Could you check a few things on this model? Use its own coordinates, in mm. Give positions to 0.01 mm unless a question says otherwise; leave off trailing zeros. Loops run counter-clockwise (first coordinate to the right, second up) from the corner with the lowest first, then second, coordinate; pieces in that order, holes last. Notation, with made-up numbers: (8, 40) - (15, 40) arc R27 cw to (15, 77) - close; hole circle Ø1 at (-22.5, 88). An arc over 180 degrees is marked (long way). Use CSV: the item, a comma, the result in double quotes.
Autodesk Inventor part; units mm, degrees
ref_plane "YZ Plane" through (0, 0, 0) normal (1, 0, 0) x (0, 1, 0)
ref_plane "XZ Plane" through (0, 0, 0) normal (0, 1, 0) x (-1, 0, 0)
ref_plane "XY Plane" through (0, 0, 0) normal (0, 0, 1) x (1, 0, 0)
sketch "スケッチ3" plane through (0, 0, 0) normal (0, 0, 1) x (1, 0, 0)
  line L0 (60, -99.3436) -> (-60, -99.3436)
  line L1 (-60, -99.3436) -> (-60, 99.3436)
  line L2 (-60, 99.3436) -> (60, 99.3436)
  line L3 (60, 99.3436) -> (60, -99.3436)
  line L4 (60, -99.3436) -> (-60, 99.3436) construction
  line L5 (-60, -99.3436) -> (60, 99.3436) construction
  point P0 (0, 0)
  dimension "d25" = 120
extrude "押し出し1" add sketch "スケッチ3" against normal blind 3
sketch "スケッチ4" plane through (0, 0, 0) normal (0, 0, 1) x (1, 0, 0)
  line L0 (0, 45.0711) -> (68.3595, 45.0711)
  line L1 (68.3595, 45.0711) -> (-74.3824, 45.0711)
  line L2 (-74.3824, 45.0711) -> (108.1656, 45.0711)
  line L3 (108.1656, 45.0711) -> (108.1656, 129.4154)
  line L4 (108.1656, 129.4154) -> (-74.3824, 129.4154)
  line L5 (-74.3824, 129.4154) -> (-74.3824, 45.0711)
  point P0 (0, 0)
extrude "押し出し4" cut sketch "スケッチ4" against normal blind 10
sketch "スケッチ13" plane through (0, 0, 0) normal (0, 0, 1) x (1, 0, 0)
  circle A0 centre (0, 0) radius 7.5
  circle A1 centre (0, 0) radius 32.5
  circle A2 centre (31.7707, 6.8465) radius 25
  circle A3 centre (31.7707, 6.8465) radius 7.5
  circle A4 centre (31.7707, 6.8465) radius 32.5
  circle A5 centre (28.5436, -25.4929) radius 25
  circle A6 centre (28.5436, -25.4929) radius 20
  circle A7 centre (28.5436, -25.4929) radius 60
  circle A8 centre (0, -78.2685) radius 40
  circle A9 centre (0, -78.2685) radius 50
  circle A10 centre (31.7707, 6.8465) radius 5.05
  circle A11 centre (28.5436, -25.4929) radius 9.55
  circle A12 centre (0, -78.2685) radius 9.55
  dimension "d87" = 65
  dimension "d89" = 65
  dimension "d91" = 120
  dimension "d86" = 15
  dimension "d88" = 15
  dimension "d90" = 40
  dimension "d92" = 100
  dimension "d96" = 10.1
  dimension "d97" = 19.1
  dimension "d98" = 19.1
extrude "押し出し16" cut sketch "スケッチ13" against normal blind 10 contours A10 A1 | A1 A10 | A11 A1 A2 | A2 A1 A4 A11 | A4 A1 A11 | A2 A11 A4 A1 | A1 A11 A2 | A4 A11 A1 | A12 A7 | A7 A12
sketch "スケッチ14" plane through (0, 0, 0) normal (0, 0, 1) x (1, 0, 0)
  point P0 (0, 0)
sketch "スケッチ15" plane through (0, 0, 0) normal (0, 0, 1) x (1, 0, 0)
  line L0 (-60, -99.3436) -> (-60, 45.0711)
  line L1 (60, 45.0711) -> (60, -99.3436)
  line L2 (-60, 45.0711) -> (60, 45.0711)
  line L3 (60, 45.0711) -> (60, -92.9289)
  line L4 (60, -92.9289) -> (-60, -92.9289)
  line L5 (-60, -92.9289) -> (-60, 45.0711)
  point P0 (0, 0)
  dimension "d101" = 138
extrude "押し出し17" cut sketch "スケッチ15" against normal blind 10 keep common part
sketch "スケッチ16" plane through (-60, 45.0711, 0) normal (0, 1, 0) x (1, 0, 0)
  line L0 (-11.4218, 21.1899) -> (145.405, 21.1899)
  line L1 (145.405, 21.1899) -> (145.405, -40.3361)
  line L2 (145.405, -40.3361) -> (-11.4218, -40.3361)
  line L3 (-11.4218, -40.3361) -> (-11.4218, 21.1899)
  point P0 (60, 0)
extrude "押し出し18" cut sketch "スケッチ16" against normal blind 10
sketch "スケッチ17" plane through (0, 0, 0) normal (0, 0, 1) x (1, 0, 0)
  circle A0 centre (31.7707, 6.8465) radius 5
  circle A1 centre (31.7707, 6.8465) radius 25
  circle A2 centre (28.5436, -25.4929) radius 9.5
  circle A3 centre (28.5436, -25.4929) radius 25
  circle A4 centre (55, -13) radius 2.1
  circle A5 centre (-55, -13) radius 2.1
  circle A6 centre (0, 29) radius 2.1
  point P0 (0, 0)
  point P1 (0, 0)
  dimension "d106" = 50
  dimension "d107" = 50
  dimension "d108" = 4.2
  dimension "d109" = 4.2
  dimension "d110" = 4.2
extrude "押し出し19" cut sketch "スケッチ17" against normal blind 10 contours A4 | A5 | A6
sketch "スケッチ18" plane through (0, 0, -3) normal (0, 0, -1) x (-1, 0, 0)
  circle A0 centre (52.5, -85.929) radius 1.6
  circle A1 centre (52.5, -77.929) radius 1.6
  circle A2 centre (-52.5, -77.929) radius 1.6
  circle A3 centre (-52.5, -85.929) radius 1.6
  point P0 (0, 0)
  dimension "d113" = 3.2
  dimension "d114" = 3.2
  dimension "d115" = 3.2
  dimension "d116" = 3.2
extrude "押し出し20" cut sketch "スケッチ18" against normal blind 10
fillet "フィレット2" radius 2 4 edges at (0, 35.0711, -3) (-60, 35.0711, -1.5) (-60, -92.9289, -1.5) (60, -92.9289, -1.5)
fillet "フィレット3" radius 2 8 edges at (60, 34.4853, -2.4142) (60, -28.9289, -3) (59.4142, -92.3431, -3) (0, -92.9289, -3) (-59.4142, -92.3431, -3) (-60, -28.9289, -3) (-59.4142, 34.4853, -2.4142) (60, 35.0711, -0.5)
properties part number "板2" material "アルミニウム 6061"
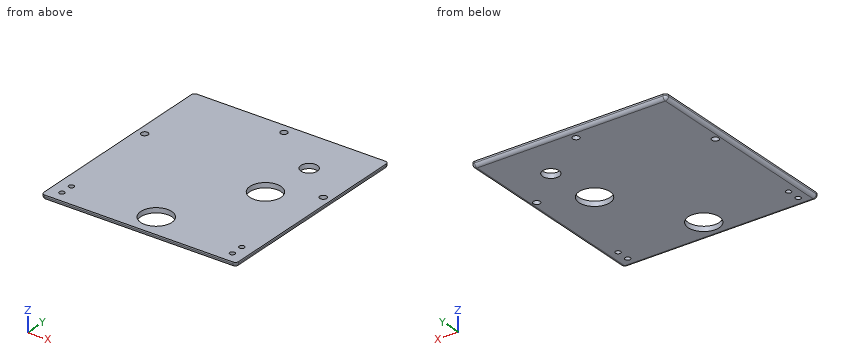
1) I'm going to push flat-ended pins straight in: P1, Ø4, axis at x = 52.5, y = -77.929, coming from the -Z side; P2, Ø2.5, axis at x = 52.5, y = -85.929, coming from the +Z side. Where does each tip first touch, or does it pass through?
Answer below:
P1,"stops at z = -3"
P2,"passes through"
2) Suppose I cut it at C-C (x = 28.5). Please give me the cut outline in (y, z).
Answer below:
outline,"(-92.93, -1) arc R2 ccw to (-90.93, -3) - (-35.04, -3) - (-35.04, 0) - (-92.93, 0) - close; (-15.94, -3) - (3, -3) - (3, 0) - (-15.94, 0) - close; (10.69, -3) - (33.07, -3) arc R2 ccw to (35.07, -1) - (35.07, 0) - (10.69, 0) - close"
3) I need wall thicknesses on line 1 along Y through (x, z) = (52.5, -1.2); line 2 along Y through (x, z) = (-55, -1); line 3 along Y through (x, z) = (52.5, -2.15). Which ranges of each line are inside material? Lowest first, please.
Answer below:
line 1,"y = -92.92 to -87.53, -84.33 to -79.53, -76.33 to 35.06"
line 2,"y = -92.93 to -15.1, -10.9 to 35.07"
line 3,"y = -92.57 to -87.53, -84.33 to -79.53, -76.33 to 34.71"
4) Suppose I cut it at A-A (y = -13). Please give me the cut outline in (x, z).
Answer below:
outline,"(-60, -1) arc R2 ccw to (-58, -3) - (-57.1, -3) - (-57.1, 0) - (-60, 0) - close; (-52.9, -3) - (52.9, -3) - (52.9, 0) - (-52.9, 0) - close; (57.1, -3) - (58, -3) arc R2 ccw to (60, -1) - (60, 0) - (57.1, 0) - close"
5) Suppose I cut it at D-D (z = -1.5). State how many separate pieces and enclosed holes the cut face has, plus the area to 3 significant figures.
Answer below:
separate pieces,"1"
enclosed holes,"10"
area,"14,600 mm2"
6) Suppose I cut it at B-B (y = 29). Please give me the cut outline in (x, z), plus the area to 3 significant figures.
Answer below:
outline,"(-60, -1) arc R2 ccw to (-58, -3) - (-2.1, -3) - (-2.1, 0) - (-60, 0) - close; (2.1, -3) - (58, -3) arc R2 ccw to (60, -1) - (60, 0) - (2.1, 0) - close"
area,"346 mm2"
